```python
from build123d import *

# Parameters (mm, degrees)
PAD_DEPTH       = 20
POCKET_DEPTH    = 18
SKETCH005_R     = 1.2
POCKET003_DEPTH = 20.001
POCKET004_DEPTH = 5
POCKET005_DEPTH = 5


with BuildPart() as part:
    # Sketch001 → Pad (new body)
    with BuildSketch(Plane.XY):
        with BuildLine():
            Line((-67.426499, 58.585), (27.6535, 58.585))
            ThreePointArc((32.698116, 58.172721), (30.184217, 58.481759), (27.6535, 58.585))
            Line((32.698116, 58.172721), (67.893206, 52.473431))
            ThreePointArc((72.6, 47.295321), (71.258477, 50.804149), (67.893206, 52.473431))
            Line((72.6, 47.295321), (72.6, -28.937809))
            ThreePointArc((67.878753, -33.701756), (71.12035, -32.19286), (72.6, -28.937809))
            Line((67.878753, -33.701756), (50.609101, -35.095512))
            Line((42.845448, -47.852044), (50.609101, -35.095512))
            ThreePointArc((38.559931, -50.255), (41.007059, -49.596346), (42.845448, -47.852044))
            Line((22.7635, -50.255), (38.559931, -50.255))
            ThreePointArc((18.35348, -49.643055), (20.537362, -50.101284), (22.7635, -50.255))
            Line((2.999306, -45.370847), (18.35348, -49.643055))
            ThreePointArc((2.999306, -45.370847), (1.67385, -45.096885), (0.3235, -45.005))
            Line((-14.8965, -45.005), (0.3235, -45.005))
            ThreePointArc((-14.8965, -45.005), (-16.054737, -45.11454), (-17.171903, -45.439275))
            Line((-49.26854, -58.28994), (-17.171903, -45.439275))
            ThreePointArc((-55.670661, -56.084897), (-52.881781, -58.384143), (-49.26854, -58.28994))
            Line((-55.670661, -56.084897), (-69.279896, -32.511389))
            Line((-69.279896, -32.511389), (-71.638452, -27.473846))
            ThreePointArc((-72.5865, -23.314273), (-72.342256, -25.446431), (-71.638452, -27.473846))
            Line((-72.5865, -23.314273), (-72.5865, 53.425))
            ThreePointArc((-67.426499, 58.585), (-71.075171, 57.073671), (-72.5865, 53.425))
        make_face()
    extrude(amount=-PAD_DEPTH)

    # Sketch002 → Pocket (cut)
    with BuildSketch(Plane.XY):
        with BuildLine():
            Line((-67.4265, 55.585), (27.6535, 55.585))
            ThreePointArc((32.06601, 55.236001), (29.866645, 55.497614), (27.6535, 55.585))
            Line((32.06601, 55.236001), (67.545103, 49.490722))
            ThreePointArc((69.6, 47.317506), (69.009594, 48.817361), (67.545103, 49.490722))
            Line((69.6, 47.317506), (69.6, -28.805775))
            ThreePointArc((67.634813, -30.711689), (68.959166, -30.11112), (69.6, -28.805775))
            Line((67.634813, -30.711689), (48.91361, -32.222593))
            ThreePointArc((48.91361, -32.222593), (48.852847, -32.240442), (48.807734, -32.284889))
            Line((40.308987, -46.249261), (48.807734, -32.284889))
            ThreePointArc((38.508222, -47.255), (39.536447, -46.98103), (40.308987, -46.249261))
            Line((22.7635, -47.255), (38.508222, -47.255))
            ThreePointArc((19.164322, -46.754702), (20.946609, -47.129327), (22.7635, -47.255))
            Line((3.804006, -42.480786), (19.164322, -46.754702))
            ThreePointArc((3.804006, -42.480786), (2.079938, -42.124497), (0.3235, -42.005))
            Line((-14.8965, -42.005), (0.3235, -42.005))
            ThreePointArc((-14.8965, -42.005), (-16.647117, -42.1735), (-18.333455, -42.672814))
            Line((-50.407295, -55.514352), (-18.333455, -42.672814))
            ThreePointArc((-53.07254, -54.584974), (-51.912632, -55.544969), (-50.407295, -55.514352))
            Line((-53.07254, -54.584974), (-66.617474, -31.122847))
            Line((-66.617474, -31.122847), (-68.929488, -26.184711))
            ThreePointArc((-69.5865, -23.291347), (-69.418415, -24.774457), (-68.929488, -26.184711))
            Line((-69.5865, -23.291347), (-69.5865, 53.425))
            ThreePointArc((-67.4265, 55.585), (-68.953851, 54.952351), (-69.5865, 53.425))
        make_face()
    extrude(amount=-POCKET_DEPTH, mode=Mode.SUBTRACT)

    # Sketch005 → Pocket003 (cut, through all)
    with BuildSketch(Plane.XY):
        with Locations((-27.0865, 32.315)):
            Circle(SKETCH005_R)
        with Locations((48.9135, -8.415)):
            Circle(SKETCH005_R)
        with Locations((48.9135, 30.085)):
            Circle(SKETCH005_R)
        with Locations((-27.0865, -5.715)):
            Circle(SKETCH005_R)
        with Locations((-51.5865, -22.915)):
            Circle(SKETCH005_R)
    extrude(amount=-POCKET003_DEPTH, mode=Mode.SUBTRACT)

    # Sketch003 (on Face7 of Pocket) → Pocket004 (cut)
    with BuildSketch(Plane(origin=(0, 58.585, 0), x_dir=(-1, 0, 0), z_dir=(0, 1, 0))):
        with BuildLine():
            Line((50.59, -4), (61.59, -4))
            ThreePointArc((63.59, -6), (63.004214, -4.585786), (61.59, -4))
            Line((63.59, -6), (63.59, -14))
            ThreePointArc((61.59, -16), (63.004214, -15.414214), (63.59, -14))
            Line((61.59, -16), (50.59, -16))
            ThreePointArc((48.59, -14), (49.175786, -15.414214), (50.59, -16))
            Line((48.59, -14), (48.59, -6))
            ThreePointArc((50.59, -4), (49.175786, -4.585786), (48.59, -6))
        make_face()
    extrude(amount=-POCKET004_DEPTH, mode=Mode.SUBTRACT)

    # Sketch004 (on Face1 of Pocket004) → Pocket005 (cut)
    with BuildSketch(Plane(origin=(-72.5865, 0, 0), x_dir=(0, -1, 0), z_dir=(-1, 0, 0))):
        with BuildLine():
            Line((-9.69, -4), (-1.69, -4))
            ThreePointArc((0.31, -6), (-0.275786, -4.585786), (-1.69, -4))
            Line((0.31, -6), (0.31, -14))
            ThreePointArc((-1.69, -16), (-0.275786, -15.414214), (0.31, -14))
            Line((-1.69, -16), (-9.69, -16))
            ThreePointArc((-11.69, -14), (-11.104214, -15.414214), (-9.69, -16))
            Line((-11.69, -14), (-11.69, -6))
            ThreePointArc((-9.69, -4), (-11.104214, -4.585786), (-11.69, -6))
        make_face()
    extrude(amount=-POCKET005_DEPTH, mode=Mode.SUBTRACT)


solid = part.part
```
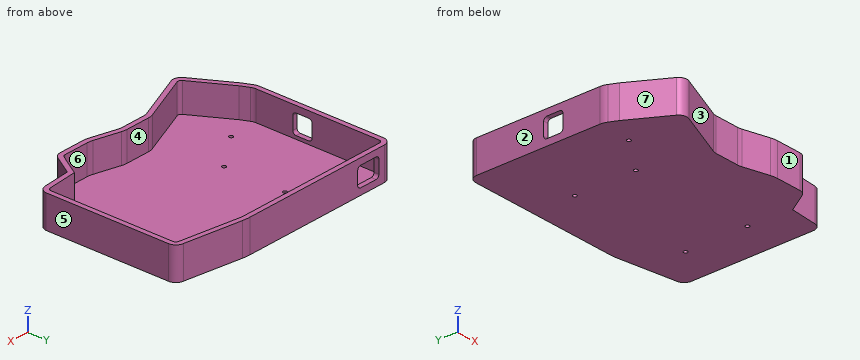
Here's how the part is built. I have some questions about the finished solid (model axes, mm). Face numbers are marked on the shaded views. A direction names the side the tool comes from. Give positions to 0.01 mm unless a question says otherwise; leave off trailing zeros. Write each loop counter-clockwise with the first axis right and the second up, starting at its lowest first coordinate (ties: lowest second). Pieces come first, ordered by that corner, then holes.
(1) If I drill on L1, parallel to X at y = -9, z = -1.75; L2, parallel to Z at x = 57, y = 9.5; L3, parallel to Y at x = -24.5, z = -10.5 (3 decimals), over which ranges is the centre line in solid material (lowest first)?
Output values:
L1: x = -72.59 to -69.59, 69.6 to 72.6
L2: z = -20 to -18
L3: y = -48.373 to -45.142, 55.585 to 58.585
(2) Imagine slicing it at A-A, the plane x = -3. Write out the boundary of the cut face in (y, z) (3 decimals), and give its area (3 significant figures).
Output values:
outline: (-45.005, -20) - (58.585, -20) - (58.585, 0) - (55.585, 0) - (55.585, -18) - (-42.005, -18) - (-42.005, 0) - (-45.005, 0) - close
area: 315 mm2
(3) On a 3-axis mill with a long thin cutter (end or side, diameter ignored), from which of +Z, -Z, +X, -X, +Y, -Y can I reach the whole of each face in a straight line? I mean the marked faces 1, 2, 3 and 4. Say none if no direction works.
Output values:
face 1: +Z, -Z, +X, -Y
face 2: +Z, -Z, -X, +Y, -Y
face 3: +Z, -Z, -Y
face 4: +Z
(4) Will these pins go through, and if not, where does the flat tip stop? pin 1 (12 mm diameter, centred on x = -4.5, z = -14, fed in from -Y); pin 2 (4.5 mm diameter, centred on x = 33, z = -11.5, fed in from -Y) (3 decimals); pin 3 (4 mm diameter, centred on x = 31.5, z = -10.5, fed in from +Y).
Output values:
pin 1: stops at y = -45.07
pin 2: stops at y = -50.255
pin 3: stops at y = 58.53
(5) Thinking about a two-plate mould opening in X: for the marked faces 5, 6 and 7, which applies, pulls with the +X half, pulls with the -X half, needs draft (parallel to the pull), parting line crosses it, or undercut?
Output values:
face 5: pulls with the +X half
face 6: undercut
face 7: pulls with the -X half
(6) Imagine slicing it at B-B, the plane y = 26. Write out the boundary of the cut face in (x, z).
Output values:
outline: (-72.59, -20) - (72.6, -20) - (72.6, 0) - (69.6, 0) - (69.6, -18) - (-69.59, -18) - (-69.59, 0) - (-72.59, 0) - close
